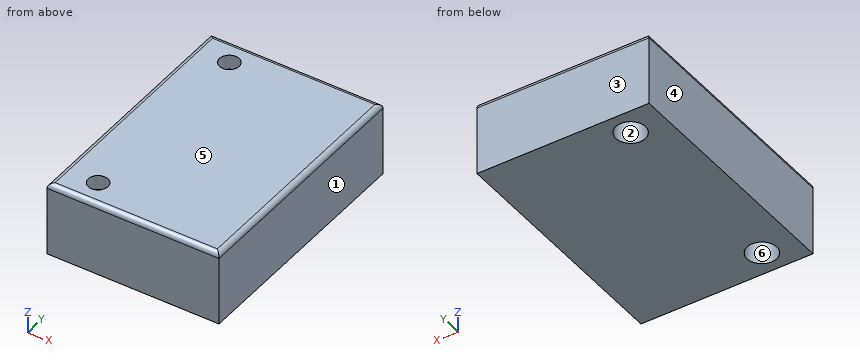
Autodesk Inventor part; units mm, degrees
ref_plane "YZ Plane" through (0, 0, 0) normal (1, 0, 0) x (0, 1, 0)
ref_plane "XZ Plane" through (0, 0, 0) normal (0, 1, 0) x (-1, 0, 0)
ref_plane "XY Plane" through (0, 0, 0) normal (0, 0, 1) x (1, 0, 0)
ref_plane "Work Plane1" through (0, 0, 0) normal (0, 0, 1) x (1, 0, 0)
sketch "SKbase" plane through (0, 0, 0) normal (0, 0, 1) x (1, 0, 0)
  line L0 (15.5, 25) -> (-19.5, 25)
  line L1 (-19.5, 25) -> (-19.5, -25)
  line L2 (-19.5, -25) -> (15.5, -25)
  line L3 (15.5, -25) -> (15.5, 25)
  point P0 (0, 0)
  point P1 (15.5, 0)
  point P2 (-2, -25)
  dimension "d0" = 35
  dimension "d1" = 50
extrude "EXbase" add sketch "SKbase" along normal blind 15
sketch "Sketch2" plane through (0, 0, 15) normal (0, 0, 1) x (1, 0, 0)
  line L0 (-12.4313, 20) -> (-12.4313, 25)
  line L1 (15.5, 25) -> (-19.5, 25)
  line L2 (-12.4313, -20) -> (-12.4313, -25)
  line L3 (-19.5, -25) -> (15.5, -25)
  point P0 (0, 0)
  dimension "d6" = 40
hole "Hole1" at (-12.4313, -20, 15) at (-12.4313, 20, 15) direction (0, 0, -1) diameter 4 end through all
fillet "Fillet1" radius 1 4 edges at (15.5, 0, 15) (-2, 25, 15) (-19.5, 0, 15) (-2, -25, 15)
sketch "Sketch3" plane through (0, 0, 0) normal (0, 0, -1) x (-1, 0, 0)
  circle A0 centre (12.4313, 20) radius 2
  circle A1 centre (12.4313, -20) radius 2
  point P0 (0, 0)
hole "Hole2" at (-12.4313, 20, 0) at (-12.4313, -20, 0) direction (0, 0, 1) diameter 6 depth 12
properties part number "optoNCDT_mount"
Input: part model. Units: mm. Frame: model coordinates. Face numbers are marked on the shaded views. A direction names the side the tool comes from. Give positions to 0.01 mm unless a question says otherwise; leave off trailing zeros. Order: outer loops, then holes, each group sorted by start corner. A loop starts at its lowest first (then second) coordinate and runs counter-clockwise, first axis right, second up. Notation, with made-up numbers: (-10.75, -9.75) -> (1.25, -9.75) arc R29 ccw to (1.25, 18.25) -> close; hole circle Ø2 at (58, -36.5). An arc over 180 degrees is marked (long way). Use one line per item in the form item = value.
1) Line query: probe 1 along X at (y, z) = (-20, 12.85); probe 2 along X at (y, z) = (-20, 3); probe 3 along Y at (x, z) = (-12, 2.75). Output: solid intervals per line, ascending.
Response values:
probe_1 = -19.5 to -14.43, -10.43 to 15.5
probe_2 = -19.5 to -15.43, -9.43 to 15.5
probe_3 = -25 to -22.97, -17.03 to 17.03, 22.97 to 25
2) Mould query, pull axis X, two halves, no side actions, for the marked faces 1, 2, 3 and 4. Classes: pulls with the +X half, pulls with the -X half, needs draft (parallel to the pull), parting line crosses it, or undercut.
Response values:
face_1 = pulls with the +X half
face_2 = undercut
face_3 = needs draft
face_4 = pulls with the -X half
3) Section B-B, the plane z = 1.75. Return loops of the section in (x, y), and give its area (3 significant figures).
Response values:
outline = (-19.5, -25) -> (15.5, -25) -> (15.5, 25) -> (-19.5, 25) -> close; hole circle Ø6 at (-12.43, -20); hole circle Ø6 at (-12.43, 20)
area = 1,690 mm^2
4) Reachability of the marked faces 5 and 6 from +Z, -Z, +X, -X, +Y, -Y: full face, straight path, thin tool, end or side. Return the list, or none.
Response values:
face_5 = +Z, +X, -X, +Y, -Y
face_6 = -Z
5) First-contact query: pin 1 Ø8 at (x, y) = (-12.43, -20) entering from -Z. Flat tip, straight axial feed; report the tip coordinate or a pass-through.
Response values:
pin_1 = 0
6) Section A-A, the plane y = -20. Return loops of the section in (x, z).
Response values:
outline = (-19.5, 0) -> (-15.43, 0) -> (-15.43, 12) -> (-14.43, 12) -> (-14.43, 15) -> (-18.5, 15) arc R1 ccw to (-19.5, 14) -> close; (-10.43, 12) -> (-9.43, 12) -> (-9.43, 0) -> (15.5, 0) -> (15.5, 14) arc R1 ccw to (14.5, 15) -> (-10.43, 15) -> close
